Geometry: final body of the model. Coordinates: model frame, mm. Give positions to 0.01 mm unless a question says otherwise; leave off trailing zeros. Loops run counter-clockwise (first coordinate to the right, second up) from the corner with the lowest first, then second, coordinate; pieces in that order, holes last.
1. Section D-D, the plane z = 2. State how many separate pieces and enclosed holes the cut face has, then the cut area to 3 significant figures.
2. Section B-B, the plane x = 6. Output: boundary loops of the cut face in (y, z), then the cut area to 3 significant figures.
3. Section C-C, the plane y = 1.6. Output: boundary loops of the cut face in (x, z), then the cut area to 3 significant figures.
4. First-contact query: P1, Ø0.5, axis at x = 0, z = 6, coming from the +Y side; P2, Ø1.5, axis at x = 5, y = -0.5, coming from the +Z side; P3, Ø0.7, axis at x = 5, z = -0.5, coming from the -Y side. Flat tips, straight axial feed; report the tip coordinate or a pass-through.
5. Section A-A, the plane z = 5. Output: boundary loops of the cut face in (x, y), then the cut area to 3 significant figures.
6. Material intervals for line 1 along X through (y, z) = (2.7, 7); line 2 along Y through (x, z) = (2.75, 5.75); line 3 along Z through (x, y) = (-1, 2.4), sorted ascending.
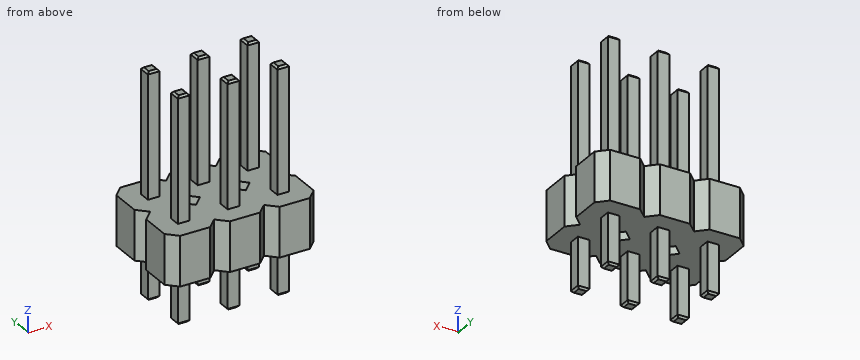
from build123d import *

# Parameters (mm, degrees)
PLASTIC_DEPTH                     = 2.54
SKETCH2_W                         = 11.44
SKETCH2_H                         = 0.6
CONTACT_DEPTH                     = 0.3
CHAMFER1_SIZE                     = 0.1
PATTERN_LINEAR_1_COUNT            = 3
PATTERN_LINEAR_1_PITCH            = 2.54
PATTERN_LINEAR_1_COUNT_DIR2       = 2
PATTERN_LINEAR_1_PITCH_DIR2       = 2.54
CHAMFER1_OF_PATTERN_LINEAR_1_SIZE = 0.1


with BuildPart() as part:
    # Sketch1 → Plastic (new body)
    with BuildSketch(Plane.XY):
        Polygon((-0.77, 1.27), (0.77, 1.27), (1.27, 0.77), (1.27, -0.77), (0.77, -1.27), (-0.77, -1.27), (-1.27, -0.77), (-1.27, 0.77), align=None)
    plastic = extrude(amount=PLASTIC_DEPTH)

    # Sketch2 → Contact (add, symmetric)
    with BuildSketch(Plane(origin=(0, 0, 0), x_dir=(0, 0, -1), z_dir=(1, 0, 0))):
        with Locations((-3.18, 0)):
            Rectangle(SKETCH2_W, SKETCH2_H)
    contact = extrude(amount=CONTACT_DEPTH, both=True)

    # Chamfer1
    chamfer1_edges = [part.edges().sort_by_distance(p)[0] for p in [
        (0, -0.3, 8.9),
        (0.3, 0, 8.9),
        (-0.3, 0, -2.54),
        (0, -0.3, -2.54),
        (0, 0.3, -2.54),
        (-0.3, 0, 8.9),
        (0, 0.3, 8.9),
        (0.3, 0, -2.54),
    ]]
    chamfer(chamfer1_edges, length=CHAMFER1_SIZE)

    # Линейный массив1: Plastic, Contact 3 × 2
    with Locations(*[(i * PATTERN_LINEAR_1_PITCH, j * PATTERN_LINEAR_1_PITCH_DIR2, 0) for i in range(PATTERN_LINEAR_1_COUNT) for j in range(PATTERN_LINEAR_1_COUNT_DIR2) if (i, j) != (0, 0)]):
        add(plastic)
        add(contact)

    # Chamfer1 of Линейный массив1
    chamfer1_of_pattern_linear_1_edges = [part.edges().sort_by_distance(p)[0] for p in [
        (0, 2.24, 8.9),
        (0.3, 2.54, 8.9),
        (-0.3, 2.54, -2.54),
        (0, 2.24, -2.54),
        (0, 2.84, -2.54),
        (-0.3, 2.54, 8.9),
        (0, 2.84, 8.9),
        (0.3, 2.54, -2.54),
        (2.54, -0.3, 8.9),
        (2.84, 0, 8.9),
        (2.24, 0, -2.54),
        (2.54, -0.3, -2.54),
        (2.54, 0.3, -2.54),
        (2.24, 0, 8.9),
        (2.54, 0.3, 8.9),
        (2.84, 0, -2.54),
        (2.54, 2.24, 8.9),
        (2.84, 2.54, 8.9),
        (2.24, 2.54, -2.54),
        (2.54, 2.24, -2.54),
        (2.54, 2.84, -2.54),
        (2.24, 2.54, 8.9),
        (2.54, 2.84, 8.9),
        (2.84, 2.54, -2.54),
        (5.08, -0.3, 8.9),
        (5.38, 0, 8.9),
        (4.78, 0, -2.54),
        (5.08, -0.3, -2.54),
        (5.08, 0.3, -2.54),
        (4.78, 0, 8.9),
        (5.08, 0.3, 8.9),
        (5.38, 0, -2.54),
        (5.08, 2.24, 8.9),
        (5.38, 2.54, 8.9),
        (4.78, 2.54, -2.54),
        (5.08, 2.24, -2.54),
        (5.08, 2.84, -2.54),
        (4.78, 2.54, 8.9),
        (5.08, 2.84, 8.9),
        (5.38, 2.54, -2.54),
    ]]
    chamfer(chamfer1_of_pattern_linear_1_edges, length=CHAMFER1_OF_PATTERN_LINEAR_1_SIZE)


solid = part.part
Answers below:
1. separate pieces: 1
1. enclosed holes: 2
1. area: 35.7 mm2
2. outline: (-1.12, 0) - (1.12, 0) - (1.12, 2.54) - (-1.12, 2.54) - close; (1.42, 0) - (3.66, 0) - (3.66, 2.54) - (1.42, 2.54) - close
2. area: 11.4 mm2
3. outline: (-1.1, 0) - (1.1, 0) - (1.1, 2.54) - (-1.1, 2.54) - close; (1.44, 0) - (3.64, 0) - (3.64, 2.54) - (1.44, 2.54) - close; (3.98, 0) - (6.18, 0) - (6.18, 2.54) - (3.98, 2.54) - close
3. area: 16.8 mm2
4. P1: stops at y = 2.84
4. P2: stops at z = 8.9
4. P3: stops at y = -0.3
5. outline: (-0.3, -0.3) - (0.3, -0.3) - (0.3, 0.3) - (-0.3, 0.3) - close; (-0.3, 2.24) - (0.3, 2.24) - (0.3, 2.84) - (-0.3, 2.84) - close; (2.24, -0.3) - (2.84, -0.3) - (2.84, 0.3) - (2.24, 0.3) - close; (2.24, 2.24) - (2.84, 2.24) - (2.84, 2.84) - (2.24, 2.84) - close; (4.78, -0.3) - (5.38, -0.3) - (5.38, 0.3) - (4.78, 0.3) - close; (4.78, 2.24) - (5.38, 2.24) - (5.38, 2.84) - (4.78, 2.84) - close
5. area: 2.16 mm2
6. line 1: x = -0.3 to 0.3, 2.24 to 2.84, 4.78 to 5.38
6. line 2: y = -0.3 to 0.3, 2.24 to 2.84
6. line 3: z = 0 to 2.54
